Answer from the drawing. Dimensions are ordinates in mm from the lowest x, y and z of the part. A direction names the side the tool comes from. Round coordinates to 2 decimals unless told otherwise and drop trailing zeros. Order: outer loops, then holes, each group sorted by start corner. A loop starts at its lowest first (then second) coordinate and runs counter-clockwise, first axis right, second up. Notation, with made-up numbers: (88, -40) -> (112, -40) arc R18 ccw to (112, -35) -> close; hole circle Ø8 at (8, 83.5). An arc over 180 degrees is marked (long way). Use a Markdown table: item, result. Add a question column.
1. Section D-D, the plane x = 2 is taken. Give the vertices of the cut face in (y, z).
2. For the marked faces 1 and 2, determine the directions among +Z, -Z, +X, -X, +Y, -Y from which every point of the face is accessible in a straight line to the end or side of a thin tool.
3. Given pin 1 (3 mm diameter, centred on y = 8, z = 1.5, fed in from +X); pin 2 (2 mm diameter, centred on y = 20, z = 8.5, fed in from +X); pin 3 (3 mm diameter, centred on x = 8.5, y = 34.5, fed in from +Z), each flat-ended and moving along its own axis, determine where each tip first touches the part or whether it passes through.
4. Consider L1, parallel to X at y = 36.5, z = 5.25; L2, parallel to Y at x = 4, z = 0.5; L3, parallel to X at y = 15.5, z = 8.75. Determine where each line is inside the solid, lowest interval first. Write a range as [from, to].
5. Section A-A, the plane x = 5.08 is taken. Give the vertices of the cut face in (y, z).
6. Section C-C, the plane z = 7.5 is taken. Give the vertices of the cut face in (x, y), then the cut area to 3 significant figures.
7. Section B-B, the plane y = 39 is taken. Give the vertices of the cut face in (x, z).
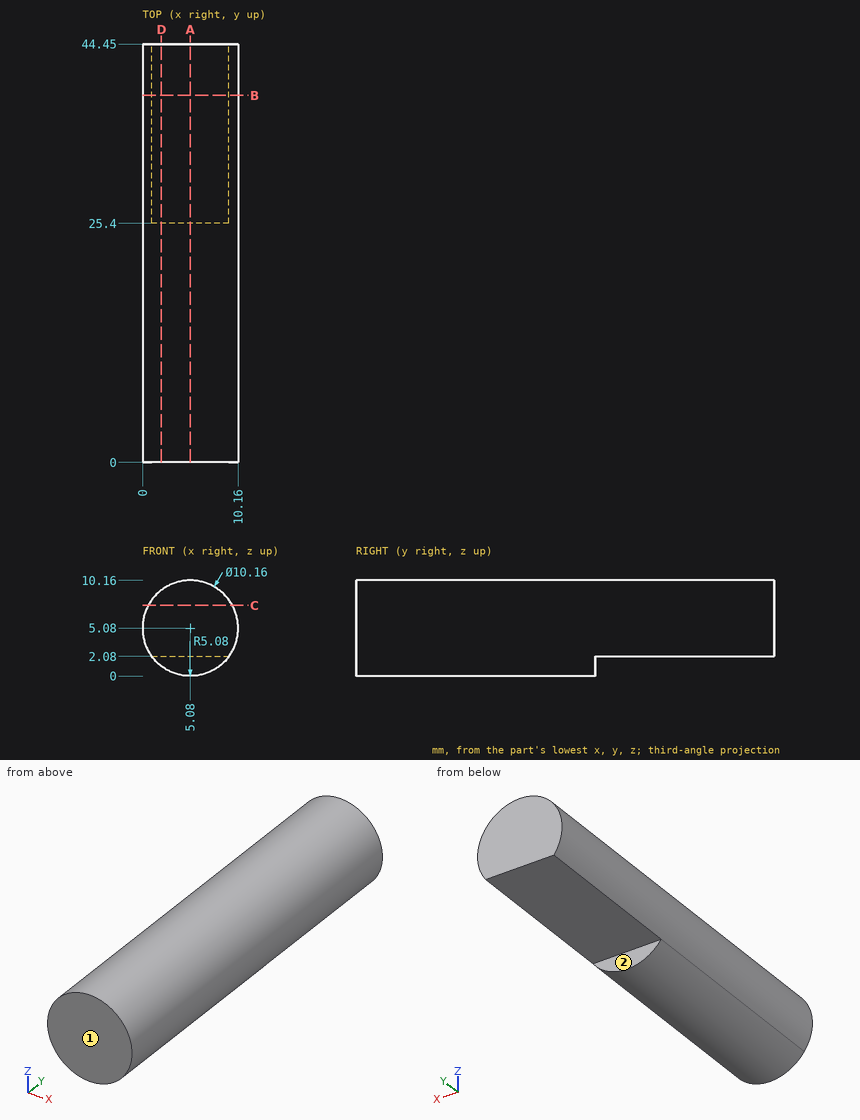
Verdict:
| question | item | result |
|---|---|---|
| 1 | outline | (0, 1.04) -> (25.4, 1.04) -> (25.4, 2.08) -> (44.45, 2.08) -> (44.45, 9.12) -> (0, 9.12) -> close |
| 2 | face 1 | +Z, -Z, +X, -X, -Y |
| 2 | face 2 | -Z, +X, -X, +Y |
| 3 | pin 1 | stops at x = 9.71 |
| 3 | pin 2 | stops at x = 9.55 |
| 3 | pin 3 | stops at z = 9.78 |
| 4 | L1 | x = [0, 10.16] |
| 4 | L2 | y = [0, 25.4] |
| 4 | L3 | x = [1.57, 8.59] |
| 5 | outline | (0, 0) -> (25.4, 0) -> (25.4, 2.08) -> (44.45, 2.08) -> (44.45, 10.16) -> (0, 10.16) -> close |
| 6 | outline | (0.61, 0) -> (9.55, 0) -> (9.55, 44.45) -> (0.61, 44.45) -> close |
| 6 | area | 397 mm2 |
| 7 | outline | (0.98, 2.08) -> (9.18, 2.08) arc R5.08 ccw (long way) to start |
